Build history of the part. All positions in model axes, mm. Face numbers are marked on the shaded views. Round coordinates to 2 decimals unless told otherwise and drop trailing zeros. Order: outer loops, then holes, each group sorted by start corner. A loop starts at its lowest first (then second) coordinate and runs counter-clockwise, first axis right, second up. Notation, with made-up numbers: (-24, 72.25) -> (17, 72.25) arc R23 cw to (17, 108.25) -> close; hole circle Ø5 at (88.5, 27.25). An arc over 180 degrees is marked (long way). Use a Markdown table: item, result. Add a question column.
Item 1: Pin check, flat tips, straight feed: pin 1 (4 mm diameter, centred on x = 25, y = 0, fed in from +Z); pin 2 (1 mm diameter, centred on x = 38.5, z = 7, fed in from +Y); pin 3 (3 mm diameter, centred on x = 38, z = 7, fed in from -Y); pin 4 (4 mm diameter, centred on y = -22, z = 12.5, fed in from +X). Stop position of each tip, or through.
Item 2: Slice it at C-C, the plane z = 3.75. Give the cut face in (x, y) (3 decimals).
Item 3: Two-plate mould, pull along Z, no slides. Class the marked faces 1, 2, 3 and 4: released by +Z, released by -Z, zero draft, split by the parting line, or undercut.
Item 4: Slice it at D-D, the plane y = 25. Give the cut face in (x, z).
Item 5: Probe L1, parallel to Y at x = 0, z = 9.75 (3 decimals); L2, parallel to Z at x = 29, y = 38.5; L3, parallel to X at y = 40, z = 1.75. List the from-to ranges inside material, lowest first.
Item 6: Slice it at A-A, the plane y = 0. Give the cut face in (x, z) (3 decimals), plus the area to 3 significant figures.
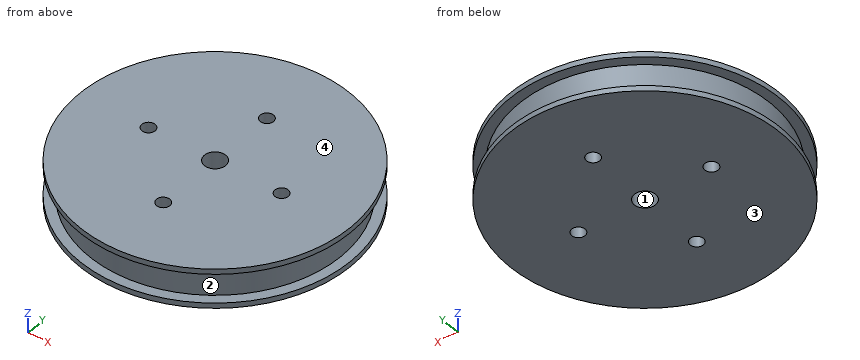
from build123d import *

# Parameters (mm, degrees)
SKETCH_1_R            = 51
SKETCH_1_R_2          = 4
EXTRUDE_1_DEPTH       = 15
HOLE_WIZARD_5_0_5_1_D = 5
CUT_EXTRUDE_START     = -13
SKETCH_4_R            = 51
SKETCH_4_R_2          = 47.365
CUT_EXTRUDE_2_DEPTH   = 11


with BuildPart() as part:
    # 草图1 → 凸台-拉伸1 (new body)
    with BuildSketch(Plane.XY):
        Circle(SKETCH_1_R)
        Circle(SKETCH_1_R_2, mode=Mode.SUBTRACT)
    extrude(amount=EXTRUDE_1_DEPTH)

    # Ø5.0 (5) 直径孔1 (through all)
    with Locations(Plane.XY.offset(15)):
        with Locations((25, 0), (0, 25), (-25, 0), (0, -25)):
            Hole(HOLE_WIZARD_5_0_5_1_D / 2)

    # 草图4 → 切除-拉伸2 (cut)
    with BuildSketch(Plane.XY.offset(15).offset(CUT_EXTRUDE_START)):
        Circle(SKETCH_4_R)
        Circle(SKETCH_4_R_2, mode=Mode.SUBTRACT)
    extrude(amount=CUT_EXTRUDE_2_DEPTH, mode=Mode.SUBTRACT)


solid = part.part
Check sheet entries:
| question | item | result |
|---|---|---|
| 1 | pin 1 | through |
| 1 | pin 2 | y = 28.27 |
| 1 | pin 3 | y = -30.19 |
| 1 | pin 4 | x = 46.89 |
| 2 | outline | circle Ø94.73 at (0, 0); hole circle Ø5 at (-25, 0); hole circle Ø8 at (0, 0); hole circle Ø5 at (0, -25); hole circle Ø5 at (0, 25); hole circle Ø5 at (25, 0) |
| 3 | face 1 | zero draft |
| 3 | face 2 | undercut |
| 3 | face 3 | released by -Z |
| 3 | face 4 | released by +Z |
| 4 | outline | (-44.45, 0) -> (-2.5, 0) -> (-2.5, 15) -> (-44.45, 15) -> (-44.45, 13) -> (-40.23, 13) -> (-40.23, 2) -> (-44.45, 2) -> close; (2.5, 0) -> (44.45, 0) -> (44.45, 2) -> (40.23, 2) -> (40.23, 13) -> (44.45, 13) -> (44.45, 15) -> (2.5, 15) -> close |
| 5 | L1 | -47.365 to -27.5, -22.5 to -4, 4 to 22.5, 27.5 to 47.365 |
| 5 | L2 | 0 to 2, 13 to 15 |
| 5 | L3 | -31.64 to 31.64 |
| 6 | outline | (-51, 0) -> (-27.5, 0) -> (-27.5, 15) -> (-51, 15) -> (-51, 13) -> (-47.365, 13) -> (-47.365, 2) -> (-51, 2) -> close; (-22.5, 0) -> (-4, 0) -> (-4, 15) -> (-22.5, 15) -> close; (4, 0) -> (22.5, 0) -> (22.5, 15) -> (4, 15) -> close; (27.5, 0) -> (51, 0) -> (51, 2) -> (47.365, 2) -> (47.365, 13) -> (51, 13) -> (51, 15) -> (27.5, 15) -> close |
| 6 | area | 1,180 mm2 |
